Can you work these out from the model? Positions are in its coordinate system, mm. Round coordinates to 2 decimals unless told otherwise and drop trailing zeros.
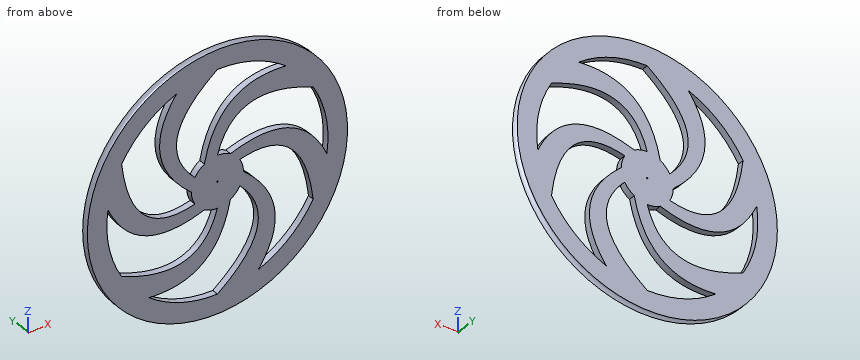
from build123d import *

# Parameters (mm, degrees)
SKETCH1_R           = 63.5
SKETCH1_R_2         = 0.3175
BOSS_EXTRUDE1_DEPTH = 3.175


with BuildPart() as part:
    # Sketch1 → Boss-Extrude1 (new body)
    with BuildSketch(Plane(origin=(0, 0, 0), x_dir=(1, 0, 0), z_dir=(0, 1, 0))):
        with Locations(Location((0, 0, 0), (0, 0, 270))):
            Circle(SKETCH1_R)
        with Locations(Location((0, 0, 0), (0, 0, 270))):
            Circle(SKETCH1_R_2, mode=Mode.SUBTRACT)
        with BuildLine():
            ThreePointArc((0, 12.7), (-3.287001873, 12.267257994), (-6.35, 10.998522628))
            add(Edge.make_bspline(
                [(-6.35, 10.998522628), (-40.0597869, 22.548298823), (-53.410384867, -7.786617578)],
                knots=[0, 0, 0, 1, 1, 1], degree=2))
            ThreePointArc((-53.410384867, -7.786617578), (-53.009631694, 10.162655788), (-46.743721169, 26.9875))
            add(Edge.make_bspline(
                [(0, 12.7), (-8.654197439, 43.517475509), (-46.743721169, 26.9875)],
                knots=[0, 0, 0, 1, 1, 1], degree=2))
        make_face(mode=Mode.SUBTRACT)
        with BuildLine():
            add(Edge.make_bspline(
                [(-10.998522628, 6.35), (-42.014338018, 14.263982923), (-46.743721169, -26.9875)],
                knots=[0, 0, 0, 1, 1, 1], degree=2))
            ThreePointArc((-10.998522628, 6.35), (-12.267257994, 3.287001873), (-12.7, 0))
            add(Edge.make_bspline(
                [(-12.7, 0), (-39.557293043, -23.418643714), (-19.961783802, -50.14805891)],
                knots=[0, 0, 0, 1, 1, 1], degree=2))
            ThreePointArc((-19.961783802, -50.14805891), (-35.305933929, -40.826359798), (-46.743721169, -26.9875))
        make_face(mode=Mode.SUBTRACT)
        with BuildLine():
            add(Edge.make_bspline(
                [(-10.998522628, -6.35), (-33.36014058, -29.253492586), (0, -53.975)],
                knots=[0, 0, 0, 1, 1, 1], degree=2))
            ThreePointArc((-10.998522628, -6.35), (-8.980256121, -8.980256121), (-6.35, -10.998522628))
            add(Edge.make_bspline(
                [(-6.35, -10.998522628), (0.502493857, -45.966942537), (33.448601066, -42.361441332)],
                knots=[0, 0, 0, 1, 1, 1], degree=2))
            ThreePointArc((33.448601066, -42.361441332), (17.703697765, -50.989015586), (0, -53.975))
        make_face(mode=Mode.SUBTRACT)
        with BuildLine():
            add(Edge.make_bspline(
                [(0, -12.7), (8.654197439, -43.517475509), (46.743721169, -26.9875)],
                knots=[0, 0, 0, 1, 1, 1], degree=2))
            ThreePointArc((0, -12.7), (3.287001873, -12.267257994), (6.35, -10.998522628))
            add(Edge.make_bspline(
                [(6.35, -10.998522628), (40.0597869, -22.548298823), (53.410384867, 7.786617578)],
                knots=[0, 0, 0, 1, 1, 1], degree=2))
            ThreePointArc((53.410384867, 7.786617578), (53.009631694, -10.162655788), (46.743721169, -26.9875))
        make_face(mode=Mode.SUBTRACT)
        with BuildLine():
            add(Edge.make_bspline(
                [(46.743721169, 26.9875), (42.014338018, -14.263982923), (10.998522628, -6.35)],
                knots=[0.554750304, 0.554750304, 0.554750304, 1.554750304, 1.554750304, 1.554750304], degree=2))
            ThreePointArc((10.998522628, -6.35), (12.267257994, -3.287001873), (12.7, 0))
            add(Edge.make_bspline(
                [(12.7, 0), (39.557293043, 23.418643714), (19.961783802, 50.14805891)],
                knots=[0, 0, 0, 1, 1, 1], degree=2))
            ThreePointArc((19.961783802, 50.14805891), (35.305933929, 40.826359798), (46.743721169, 26.9875))
        make_face(mode=Mode.SUBTRACT)
        with BuildLine():
            add(Edge.make_bspline(
                [(0, 53.975), (33.36014058, 29.253492586), (10.998522628, 6.35)],
                knots=[0.274970858, 0.274970858, 0.274970858, 1.274970858, 1.274970858, 1.274970858], degree=2))
            ThreePointArc((10.998522628, 6.35), (8.980256121, 8.980256121), (6.35, 10.998522628))
            add(Edge.make_bspline(
                [(6.35, 10.998522628), (-0.502493857, 45.966942537), (-33.448601066, 42.361441332)],
                knots=[0, 0, 0, 1, 1, 1], degree=2))
            ThreePointArc((-33.448601066, 42.361441332), (-17.703697765, 50.989015586), (0, 53.975))
        make_face(mode=Mode.SUBTRACT)
    extrude(amount=BOSS_EXTRUDE1_DEPTH)

    # Sketch2 → Cut-Revolve2 (revolve, cut)
    with BuildSketch(Plane.XY):
        with BuildLine():
            Line((-63.5, 0), (-63.5, 3.175))
            add(Edge.make_bspline(
                [(-63.5, 3.175), (-60.325, 1.5875), (-63.5, 0)],
                knots=[0, 0, 0, 1, 1, 1], degree=2))
        make_face()
    revolve(axis=Axis((0, 0, 0), (0, 1, 0)), mode=Mode.SUBTRACT)


solid = part.part
(1) Will these pins go through, and if not, where does the flat tip stop? P1, Ø3, axis at x = 26, z = 37.5, coming from the -Y side; P2, Ø1, axis at x = -31, y = 1, coming from the +Z side.
Worked answers:
P1: stops at y = 0
P2: stops at z = 54.5
(2) If I drill on line 1 (X direction, y = 2.4, z = -9); line 2 (X direction, y = 2.2, z = -34.5); line 3 (Z direction, x = -29, y = 2.5), over which ranges is the centre line in solid material (lowest first)?
Worked answers:
line 1: x = -61.68 to -53.22, -40.64 to 8.96, 13.39 to 21.21, 42.56 to 61.68
line 2: x = -51.69 to -4.93, 17.77 to 27.52, 41.51 to 51.69
line 3: z = -55.29 to -45.52, -42.68 to -32.37, -13.73 to -6.07, 45.52 to 55.29
(3) If we section it at A-A, the plane x = -44: State how many separate pieces and enclosed holes the cut face has, then the cut area to 3 significant figures.
Worked answers:
separate pieces: 3
enclosed holes: 0
area: 154 mm2
